The model under review builds one solid part; all positions refer to its coordinate system, in mm. Give positions to 0.01 mm unless a question says otherwise; leave off trailing zeros. Write each loop counter-clockwise with the first axis right and the second up, starting at its lowest first coordinate (ties: lowest second). Pieces come first, ordered by that corner, then holes. Notation, with made-up numbers: (-25.5, -27.75) - (2.5, -27.75) arc R26 cw to (2.5, 2.25) - close; hole circle Ø8 at (54.5, 20.25). An arc over 180 degrees is marked (long way). Write item = value, one per line.
Autodesk Inventor part; units mm, degrees
ref_plane "YZ Plane" through (0, 0, 0) normal (1, 0, 0) x (0, 1, 0)
ref_plane "XZ Plane" through (0, 0, 0) normal (0, 1, 0) x (-1, 0, 0)
ref_plane "XY Plane" through (0, 0, 0) normal (0, 0, 1) x (1, 0, 0)
ref_plane "Work Plane1" through (-0.1788, 0, 0) normal (0, 0, 1) x (1, 0, 0)
sketch "Sketch1" plane through (-0.1788, 0, 0) normal (0, 0, 1) x (1, 0, 0)
  line L0 (-15.3244, 3.4987) -> (-19.1223, 3.4987)
  line L1 (-19.1223, 3.4987) -> (-28.8529, 35.0248)
  arc A0 (-28.8529, 35.0248) -> (-20.5467, 47.7802) centre (-25.0147, 41.6076) ccw
  line L2 (-20.5467, 47.7802) -> (-6.566, 47.7802)
  arc A1 (-6.566, 47.7802) -> (-2.0556, 33.1897) centre (0.3832, 41.936) ccw
  line L3 (-2.0556, 33.1897) -> (-2.0556, 15.9522)
  arc A2 (-2.0556, 15.9522) -> (-15.3244, 3.4987) centre (0.3832, 0.0582) ccw
  arc A3 (20.8934, 47.7802) -> (21.5632, 35.5913) centre (25.7832, 41.936) ccw
  line L4 (21.5632, 35.5913) -> (21.5632, 4.0758)
  line L5 (21.5632, 4.0758) -> (15.9532, 4.0758)
  arc A4 (15.9532, 4.0758) -> (1.9969, 16.0571) centre (0.3832, 0.0582) ccw
  line L6 (1.9969, 16.0571) -> (1.9969, 33.0006)
  arc A5 (1.9969, 33.0006) -> (7.3324, 47.7802) centre (0.3832, 41.936) ccw
  line L7 (7.3324, 47.7802) -> (20.8934, 47.7802)
  arc A6 (21.5632, -35.3114) -> (21.3082, -47.8332) centre (25.7764, -41.6607) ccw
  line L8 (21.3082, -47.8332) -> (7.1864, -47.8332)
  arc A7 (7.1864, -47.8332) -> (1.9969, -32.8841) centre (0.3832, -41.8196) ccw
  line L9 (1.9969, -32.8841) -> (1.9969, -15.9406)
  arc A8 (1.9969, -15.9406) -> (16.068, -3.4851) centre (0.3832, 0.0582) ccw
  line L10 (16.068, -3.4851) -> (21.5632, -3.4851)
  line L11 (21.5632, -3.4851) -> (21.5632, -35.3114)
  arc A9 (-20.9828, -47.8332) -> (-29.9021, -35.476) centre (-25.464, -41.6702) ccw
  line L12 (-29.9021, -35.476) -> (-19.2115, -3.4851)
  line L13 (-19.2115, -3.4851) -> (-15.3016, -3.4851)
  arc A10 (-15.3016, -3.4851) -> (-2.0556, -15.8358) centre (0.3832, 0.0582) ccw
  line L14 (-2.0556, -15.8358) -> (-2.0556, -33.0732)
  arc A11 (-2.0556, -33.0732) -> (-6.4199, -47.8332) centre (0.3832, -41.8196) ccw
  line L15 (-6.4199, -47.8332) -> (-20.9828, -47.8332)
  circle A12 centre (0.3832, 0.0582) radius 11
  circle A13 centre (0.3832, -41.8196) radius 4
  circle A14 centre (0.3832, 41.936) radius 4
  circle A15 centre (-25.464, -41.6702) radius 2.54
  circle A16 centre (-25.0147, 41.6076) radius 2.54
  circle A17 centre (25.7764, -41.6607) radius 2.54
  circle A18 centre (25.7832, 41.936) radius 2.54
  arc A19 (25.7764, 31.8658) -> (25.2733, 51.9934) centre (25.7832, 41.936) ccw
  line L16 (25.2733, 51.9934) -> (-25.0147, 51.9934)
  arc A20 (-25.0147, 51.9934) -> (-35.3953, 41.9358) centre (-25.0147, 41.6076) ccw
  line L17 (-35.3953, 41.9358) -> (-22.4697, 0.058)
  line L18 (-22.4697, 0.058) -> (-35.3142, -38.3784)
  arc A21 (-35.3142, -38.3784) -> (-25.0214, -52.0464) centre (-25.464, -41.6702) ccw
  line L19 (-25.0214, -52.0464) -> (25.7764, -52.0464)
  arc A22 (25.7764, -52.0464) -> (25.7764, -31.275) centre (25.7764, -41.6607) ccw
  line L20 (25.7764, -31.275) -> (25.7764, 31.8658)
  line L21 (0.1293, 51.9934) -> (0.1293, 62.509)
  line L22 (-35.3953, 41.9358) -> (-48.0953, 41.9358)
  line L23 (-47.8239, 62.509) -> (41.0761, 62.509)
  line L24 (41.0761, 62.509) -> (110.9261, -286.741)
  line L25 (-47.8239, 62.509) -> (-47.8239, -286.741)
  line L26 (-47.8239, -286.741) -> (110.9261, -286.741)
  point P0 (0.1788, 0)
  dimension "d0" = 10.5156
  dimension "d1" = 12.7
  dimension "d4" = 88.9
  dimension "d10" = 349.25
extrude "Extrusion1" add sketch "Sketch1" along normal blind 6.096 contours L0 L1 A0 L2 A1 L3 A2 | A3 L4 L5 A4 L6 A5 L7 | A6 L8 A7 L9 A8 L10 L11 | A9 L12 L13 A10 L14 A11 L15 | A12 | L20 A22 L19 A21 L18 L17 A20 L16 A19 | A19 L16 L21 L23 L24 L26 L25 L22 L17 L18 A21 L19 A22 L20 | L16 A20 L22 L25 L23 L21
sketch "Sketch2" plane through (-0.1788, 0, 6.096) normal (0, 0, 1) x (1, 0, 0)
  circle A0 centre (0.3832, 0.0582) radius 5
  point P0 (0.1788, 0)
extrude "Extrusion2" cut sketch "Sketch2" against normal blind 25.4
sketch "Sketch3" plane through (-0.1788, 0, 0) normal (0, 0, -1) x (-1, 0, 0)
  circle A0 centre (-0.3832, 0.0582) radius 5
  circle A1 centre (-0.3832, 41.936) radius 4
  circle A2 centre (-0.3832, -41.8196) radius 4
  circle A3 centre (-25.7832, 41.936) radius 2.54
  circle A4 centre (-25.7764, -41.6607) radius 2.54
  circle A5 centre (25.0147, 41.6076) radius 2.54
  circle A6 centre (25.464, -41.6702) radius 2.54
  line L0 (47.8239, 62.509) -> (-41.0761, 62.509)
  line L1 (-41.0761, 62.509) -> (-110.9261, -286.741)
  line L2 (-110.9261, -286.741) -> (47.8239, -286.741)
  line L3 (47.8239, -286.741) -> (47.8239, 62.509)
  line L4 (82.12, -280.645) -> (-254.43, -280.645)
  line L5 (-72.5025, -280.645) -> (-68.0575, -280.645)
  line L6 (-21.7025, -280.645) -> (-17.2575, -280.645)
  line L7 (29.0975, -280.645) -> (33.5425, -280.645)
  line L8 (-70.28, -280.645) -> (-70.28, -267.945)
  line L9 (-70.28, -267.945) -> (-19.48, -267.945)
  line L10 (-19.48, -267.945) -> (31.32, -267.945)
  line L11 (31.32, -267.945) -> (31.32, -242.545)
  circle A7 centre (-70.28, -267.945) radius 2.2225
  circle A8 centre (-19.48, -267.945) radius 2.2225
  circle A9 centre (31.32, -267.945) radius 2.2225
  circle A10 centre (31.32, -242.545) radius 2.2225
  circle A11 centre (-19.48, -242.545) radius 2.2225
  circle A12 centre (-70.28, -242.545) radius 2.2225
  point P0 (-0.1788, 0)
  dimension "d11" = 12.7
  dimension "d12" = 25.4
  dimension "d13" = 4.445
  dimension "d14" = 4.445
  dimension "d15" = 4.445
  dimension "d16" = 4.445
  dimension "d17" = 4.445
  dimension "d18" = 4.445
extrude "Extrusion3" cut sketch "Sketch3" against normal blind 25.4 contours A10 | A9 L11 L10 | L10 L11 A9 | A8 L10 L9 | L9 L10 A8 | A7 L9 L8 | L8 L9 A7 | A11 | A12
sketch "Sketch4" plane through (-0.1788, 0, 0) normal (0, 0, -1) x (-1, 0, 0)
  circle A0 centre (-19.48, -242.545) radius 2.2225
  circle A1 centre (31.32, -267.945) radius 2.2225
  circle A2 centre (-70.28, -267.945) radius 2.2225
  circle A3 centre (-19.48, -267.945) radius 2.2225
  circle A4 centre (31.32, -242.545) radius 2.2225
  circle A5 centre (-70.28, -242.545) radius 2.2225
  circle A6 centre (-0.3832, 0.0582) radius 5
  circle A7 centre (-0.3832, 41.936) radius 4
  circle A8 centre (-0.3832, -41.8196) radius 4
  circle A9 centre (-25.7832, 41.936) radius 2.54
  circle A10 centre (-25.7764, -41.6607) radius 2.54
  circle A11 centre (25.0147, 41.6076) radius 2.54
  circle A12 centre (25.464, -41.6702) radius 2.54
  line L0 (47.8239, 62.509) -> (-41.0761, 62.509)
  line L1 (-41.0761, 62.509) -> (-110.9261, -286.741)
  line L2 (-110.9261, -286.741) -> (47.8239, -286.741)
  line L3 (47.8239, -286.741) -> (47.8239, 62.509)
  point P0 (-0.1788, 0)
sketch "Sketch5" plane through (-0.1788, 0, 6.096) normal (0, 0, 1) x (1, 0, 0)
  circle A0 centre (0.3832, -41.8196) radius 4
  line L0 (0.3832, -41.8196) -> (0.3832, -118.0196)
  point P0 (0.1788, 0)
  dimension "d21" = 76.2
sketch "Sketch6" plane through (-0.1788, 0, 6.096) normal (0, 0, 1) x (1, 0, 0)
  line L0 (41.0761, 62.509) -> (-47.8239, 62.509)
  line L1 (-47.8239, 62.509) -> (-47.8239, -89.891)
  line L2 (-47.8239, 62.509) -> (-47.8239, -286.741)
  line L3 (-47.8239, -89.891) -> (-28.7739, -89.891)
  line L4 (-28.7739, -89.891) -> (-28.7739, -127.991)
  circle A0 centre (-28.7739, -89.891) radius 2.2225
  circle A1 centre (-28.7739, -127.991) radius 2.2225
  point P0 (0.1788, 0)
  dimension "d22" = 152.4
  dimension "d23" = 19.05
  dimension "d24" = 38.1
  dimension "d25" = 4.445
  dimension "d26" = 4.445
extrude "Extrusion4" cut sketch "Sketch6" against normal blind 25.4
properties part number "Side Walls"
1. For line 1 (X direction, y = 3.5, z = 3.75); line 2 (X direction, y = -107.5, z = 3.5); line 3 (X direction, y = -59, z = 0.5), list the stretches that pass through material, from the lowest coordinate up. Write a range as from..to.
Findings below:
line_1 = -48..-3.42, 3.83..52.7
line_2 = -48..74.9
line_3 = -48..65.2
2. Take a section at C-C on x = 98. Give the boundary of the cut face in (y, z), and give its area (3 significant figures).
Findings below:
outline = (-286.74, 0) - (-223, 0) - (-223, 6.1) - (-286.74, 6.1) - close
area = 389 mm²
3. Take a section at A-A on z = 4.5. Count the separate pieces of the cut face and the enclosed holes in it, and give its area (3 significant figures).
Findings below:
separate_pieces = 1
enclosed_holes = 15
area = 42,900 mm²
4. Take a section at B-B on y = -32. Give the boundary of the cut face in (x, z).
Findings below:
outline = (-48, 0) - (59.8, 0) - (59.8, 6.1) - (-48, 6.1) - close
5. Draft analysis for pull direction Y (two halves, no side actions). For faces 1 (the flat face through (30, -286.741, 3)), 2 (the cylindrical face through (-0.663, -37.915, 3.005)), 3 (the flat face through (75.333, -109.671, 3.005)), state which applies: +Y half, -Y half, draft (parallel to the pull), parting line (faces both ways), or undercut.
Findings below:
face_1 = -Y half
face_2 = undercut
face_3 = +Y half
6. Insertion check: P1, Ø4, axis at x = -28.95, y = -127.99, coming from the -Z side. The pin has a flat end and moves straight along its axis. Give the tip position at first contact, or say it passes through.
Findings below:
P1 = through
